Autodesk Inventor part; units mm, degrees
ref_plane "YZ Plane" through (0, 0, 0) normal (1, 0, 0) x (0, 1, 0)
ref_plane "XZ Plane" through (0, 0, 0) normal (0, 1, 0) x (-1, 0, 0)
ref_plane "XY Plane" through (0, 0, 0) normal (0, 0, 1) x (1, 0, 0)
sketch "Schizzo1" plane through (0, 0, 0) normal (0, 1, 0) x (-1, 0, 0)
  line L0 (300, 0) -> (300, 15)
  line L1 (0, 0) -> (0, 400)
  line L2 (0, 400) -> (15, 400)
  line L3 (15, 400) -> (71.5685, 343.4315)
  line L4 (15, 400) -> (95, 400) construction
  line L5 (71.5685, 343.4315) -> (60.9619, 332.8249)
  line L6 (60.9619, 332.8249) -> (15, 378.7868)
  line L7 (15, 378.7868) -> (15, 15)
  line L8 (300, 15) -> (15, 15)
  line L9 (300, 0) -> (300, -60)
  line L10 (300, -60) -> (240, -60)
  line L11 (240, -60) -> (240, -45)
  line L12 (240, -45) -> (285, -45)
  line L13 (285, -45) -> (285, 0)
  line L14 (285, 0) -> (0, 0)
  dimension "d1" = 15
  dimension "d3" = 400
  dimension "d4" = 15
  dimension "d5" = 80
  dimension "d6" = 45
  dimension "d7" = 15
  dimension "d8" = 60
  dimension "d9" = 60
  dimension "d10" = 15
  dimension "d11" = 45
extrude "Estrusione1" add sketch "Schizzo1" along normal blind 20
equation "\"RaggioPiega\" = Spessore"
equation "\"LarghezzaScaricoPiega\" = Spessore"
equation "\"ProfonditàScaricoPiega\" = 0.5 * Spessore"
equation "\"DimensioniScaricoAngolo\" = 4 * Spessore"
equation "\"ResiduoMinimo\" = 2 * Spessore"
equation "\"RaggioTransizione\" = RaggioPiega"
equation "\"Dimensione_raggio_Jacobi\" = RaggioPiega"
equation "\"DimensioneGioco\" = Spessore"
properties part number "Staffa"
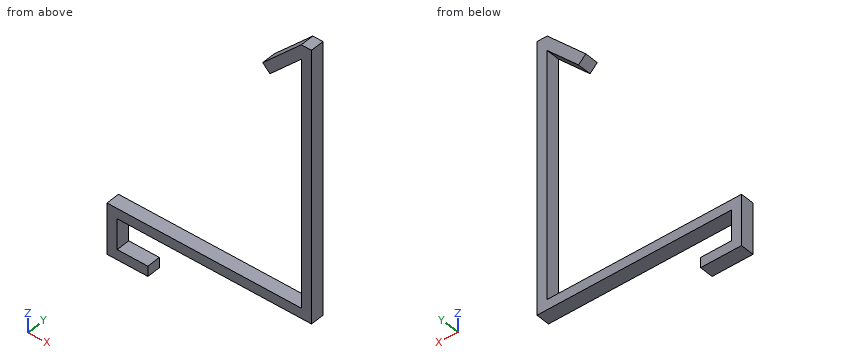
For this review, take the finished solid that the model builds, in its own axes (mm). Give positions to 0.01 mm unless a question says otherwise; leave off trailing zeros. Loops run counter-clockwise (first coordinate to the right, second up) from the corner with the lowest first, then second, coordinate; pieces in that order, holes last. Notation, with made-up numbers: M 69.25,78 L 94.25,78 A13 ccw 94.25,100 Z; hole C 5,-9.5 d5. An arc over 180 degrees is marked long. One line per item, written item: value. Start each with the question number.
Q1. Add section A-A (x = -253). Give the boundary of the cut face in (y, z).
Q2. Add section D-D (z = 185). Give the boundary of the cut face in (x, y).
Q3. For L1, parallel to Z at x = -280.5, y = 9; L2, parallel to X at y = 3.75, z = -24; L3, parallel to X at y = 8.5, z = 29, list the stretches that pass through material, from the lowest coordinate up.
Q4. Add section C-C (y = 10). Give the boundary of the cut face in (x, z).
Q5. Add section B-B (z = 367). Give the boundary of the cut face in (x, y), and give its area (3 significant figures).
Q6. Clearance check with flat-ended pins moving along their axes: pin 1 Ø10 at (x, y) = (-101, 7.5) entering from +Z; pin 2 Ø4 at (x, y) = (-41.5, 3.5) entering from +Z; pin 3 Ø1 at (x, y) = (-184, 14.5) entering from -Z. State where each tip first meets the part, or that it passes through.
Reply:
1. outline: M 0,-60 L 20,-60 L 20,-45 L 0,-45 Z; M 0,0 L 20,0 L 20,15 L 0,15 Z
2. outline: M -15,0 L 0,0 L 0,20 L -15,20 Z
3. L1: -60 to -45, 0 to 15
3. L2: -300 to -285
3. L3: -15 to 0
4. outline: M -300,-60 L -240,-60 L -240,-45 L -285,-45 L -285,0 L 0,0 L 0,400 L -15,400 L -71.57,343.43 L -60.96,332.82 L -15,378.79 L -15,15 L -300,15 Z
5. outline: M -48,0 L -26.79,0 L -26.79,20 L -48,20 Z; M -15,0 L 0,0 L 0,20 L -15,20 Z
5. area: 724 mm²
6. pin 1: z = 15
6. pin 2: z = 375.5
6. pin 3: z = 0
